Autodesk Fusion 360 part; units mm, degrees
sketch "Sketch1" plane through (0, 0, 0) normal (0, 1, 0) x (1, 0, 0)
  circle A0 centre (0, 0) radius 3
  dimension "d1" = 6
extrude "Extrude1" add sketch "Sketch1" along normal blind 91
sketch "Sketch2" plane through (0, 0, 0) normal (0, -1, 0) x (1, 0, 0)
  circle A0 centre (0, 0) radius 3
  circle A1 centre (0, 0) radius 2
  dimension "d4" = 4
extrude "Extrude2" add sketch "Sketch2" along normal blind 4 contours A1
sketch "Sketch3" plane through (0, -4, 0) normal (0, -1, 0) x (1, 0, 0)
  circle A0 centre (0, 0) radius 2
  circle A1 centre (0, 0) radius 1.5
  dimension "d7" = 3
extrude "Extrude3" add sketch "Sketch3" along normal blind 17 contours A1
chamfer "Chamfer1" distance 0.5 angle 45 1 edges at (-1.3985, -4, 0.5424)
extrude "Extrude4" cut 1 faces at (0.567, -21, -0.5383) along direction (0, 1, 0) blind 1.5
chamfer "Chamfer3" distance 1.5 angle 65 1 edges at (-1.3985, -19.5, 0.5424) measured on face at (0.567, -19.5, -0.5383)
equation "d13 = 19.5 mm - 21.00 mm"
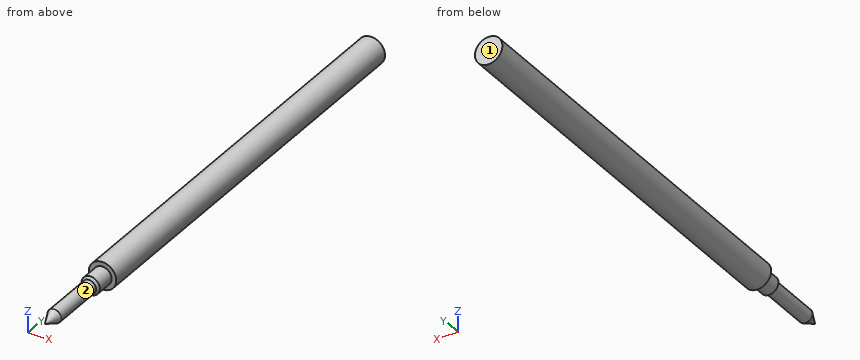
Could you check a few things on this model? Use its own coordinates, in mm. Face numbers are marked on the shaded views. A direction names the side the tool comes from. Give positions to 0.01 mm unless a question says otherwise; leave off trailing zeros. Order: outer loops, then holes, each group sorted by start corner. A loop starts at its lowest first (then second) coordinate and runs counter-clockwise, first axis right, second up. Notation, with made-up numbers: (-30, 67.5) -> (-3, 67.5) arc R26 cw to (-3, 95.5) -> close; hole circle Ø11 at (11, 29.5). An arc over 180 degrees is marked (long way). Answer in a Markdown table with one row per item. Add a question column.
Item 1: For the marked faces 1 and 2, which set-ups out of +Z, -Z, +X, -X, +Y, -Y let a thin tool reach every point of the face, with its end or its side?
Item 2: I'm going to push flat-ended pins straight in: P1, Ø1, axis at y = 66.5, z = 2, coming from the -X side; P2, Ø3, axis at x = 2, y = 63.5, coming from the -Z side; P3, Ø1.8, axis at x = -1, z = 0, coming from the -Y side. Where does each tip first touch, or does it pass through?
Item 3: Imagine slicing it at A-A (y = 9). List the corners of the cut face in (x, z) for me.
Item 4: Please list where these lines run through material, in increasing order: probe 1 along Y at (x, z) = (2.1, -1.5); probe 2 along Z at (x, y) = (0.1, 62.5); probe 3 along Z at (x, y) = (-0.9, 56).
Result:
| question | item | result |
|---|---|---|
| 1 | face 1 | +Z, -Z, +X, -X, +Y |
| 1 | face 2 | -Y |
| 2 | P1 | x = -2.6 |
| 2 | P2 | z = -2.96 |
| 2 | P3 | y = -19.29 |
| 3 | outline | circle Ø6 at (0, 0) |
| 4 | probe 1 | 0 to 91 |
| 4 | probe 2 | -3 to 3 |
| 4 | probe 3 | -2.86 to 2.86 |
